Job drawing, mm, ordinate dimensions from the low corner. One solid piece. Give positions to 0.01 mm unless a question says otherwise; leave off trailing zeros. Order: outer loops, then holes, each group sorted by start corner. A loop starts at its lowest first (then second) coordinate and runs counter-clockwise, first axis right, second up. Notation, with made-up numbers: M -19,-9.5 L 30,-9.5 A23 cw 30,11.5 Z; hole C 54,76.25 d6. An arc over 180 degrees is marked long. One line per question, with ' | ' between items.
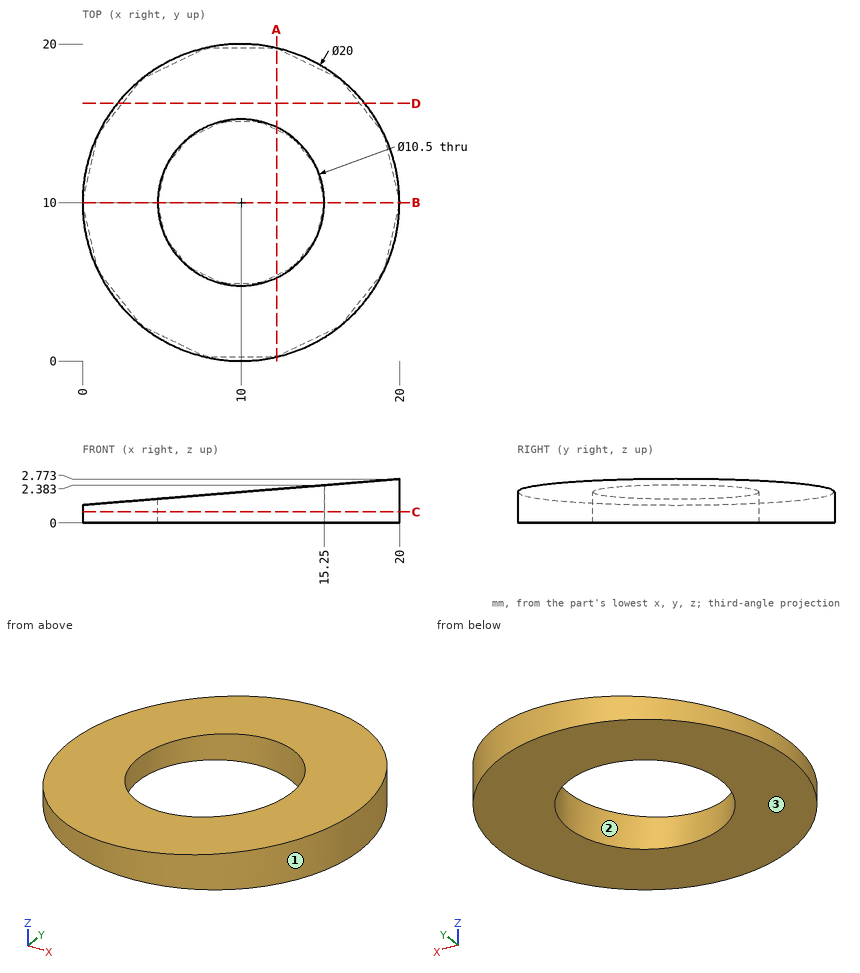
1. Drop flat-ended pins along their axis: pin 1 (2 mm diameter, centred on x = 8.5, y = 2.5, fed in from +Z); pin 2 (8.5 mm diameter, centred on x = 10, y = 10, fed in from -Z); pin 3 (1 mm diameter, centred on y = 8.5, z = 2, fed in from +X). Give the stop position or say it passes through.
Worked out:
pin 1: stops at z = 1.91 | pin 2: passes through | pin 3: stops at x = 19.95
2. Slice it at A-A on x = 12.25. Give the cut face in (y, z).
Worked out:
outline: M 0.26,0 L 5.26,0 L 5.26,2.14 L 0.26,2.14 Z; M 14.74,0 L 19.74,0 L 19.74,2.14 L 14.74,2.14 Z
3. Slice it at B-B on y = 10. Give the cut face in (x, z).
Worked out:
outline: M 0,0 L 4.75,0 L 4.75,1.52 L 0,1.13 Z; M 15.25,0 L 20,0 L 20,2.77 L 15.25,2.38 Z
4. Probe L1, parallel to Y at x = 10, z = 0.7; L2, parallel to Y at x = 14, z = 1.4 (1 decimal); L3, parallel to X at y = 10, z = 1.95. List the from-to ranges inside material, lowest first. Write a range as from..to.
Worked out:
L1: y = 0..4.75, 15.25..20 | L2: y = 0.8..6.6, 13.4..19.2 | L3: x = 15.25..20
5. Mould opens along Y. For the marked faces 1, 2 and 3 say: released by +Y, released by -Y, zero draft, split by the parting line, or undercut.
Worked out:
face 1: split by the parting line | face 2: undercut | face 3: zero draft
6. Slice it at C-C on z = 0.7. Give the cut face in (x, y).
Worked out:
outline: C 10,10 d20; hole C 10,10 d10.5
7. Slice it at D-D on y = 16.25. Give the cut face in (x, z).
Worked out:
outline: M 2.19,0 L 17.81,0 L 17.81,2.59 L 2.19,1.31 Z
